from build123d import *
from build123d.topology import SkipClean

# Parameters (mm, degrees)
SKETCH3_W           = 1.5875
SKETCH3_H           = 89.802561211
BOSS_EXTRUDE2_DEPTH = 12.7
BOSS_EXTRUDE4_DEPTH = 6.35
BOSS_EXTRUDE5_DEPTH = 12.7
BOSS_EXTRUDE6_START = -6.35
BOSS_EXTRUDE6_DEPTH = 6.35
CUT_EXTRUDE1_DEPTH  = 1.5875
SKETCH5_W           = 4.7625
SKETCH5_H           = 1.5875
BOSS_EXTRUDE7_DEPTH = 70.752561211
CUT_EXTRUDE2_DEPTH  = 12.7
FILLET1_R           = 3.175
FILLET2_R           = 3.175


# Read off the part's stored shape, not the designer's step: Mirror3
with BuildPart() as part:
    # Sketch3 → Boss-Extrude2 (new body)
    with BuildSketch(Plane(origin=(0, 0, 0), x_dir=(1, 0, 0), z_dir=(0, 1, 0))):
        with Locations((0.79375, 44.901280606)):
            Rectangle(SKETCH3_W, SKETCH3_H)
    extrude(amount=BOSS_EXTRUDE2_DEPTH)

    # Sketch4 → Boss-Extrude4 (add)
    with BuildSketch(Plane(origin=(1.5875, 0, 0), x_dir=(0, 0, -1), z_dir=(1, 0, 0))):
        with BuildLine():
            ThreePointArc((0, 0), (4.490128061, 1.859871939), (6.35, 6.35))
            ThreePointArc((6.35, 6.35), (4.490128061, 10.840128061), (0, 12.7))
            Line((0, 12.7), (0, 9.525))
            ThreePointArc((0, 9.525), (2.24506403, 8.59506403), (3.175, 6.35))
            ThreePointArc((3.175, 6.35), (2.24506403, 4.10493597), (0, 3.175))
            Line((0, 3.175), (0, 0))
        make_face()
        with BuildLine():
            Line((0, 9.525), (0, 12.7))
            ThreePointArc((0, 12.7), (-6.35, 6.35), (0, 0))
            Line((0, 0), (0, 3.175))
            ThreePointArc((0, 3.175), (-3.175, 6.35), (0, 9.525))
        make_face()
        with BuildLine():
            ThreePointArc((0, 0), (4.490128061, 1.859871939), (6.35, 6.35))
            ThreePointArc((6.35, 6.35), (4.490128061, 10.840128061), (0, 12.7))
            Line((0, 12.7), (0, 9.525))
            ThreePointArc((0, 9.525), (2.24506403, 8.59506403), (3.175, 6.35))
            ThreePointArc((3.175, 6.35), (2.24506403, 4.10493597), (0, 3.175))
            Line((0, 3.175), (0, 0))
        make_face()
        with BuildLine():
            Line((0, 9.525), (0, 12.7))
            ThreePointArc((0, 12.7), (-6.35, 6.35), (0, 0))
            Line((0, 0), (0, 3.175))
            ThreePointArc((0, 3.175), (-3.175, 6.35), (0, 9.525))
        make_face()
        with BuildLine():
            Line((6.35, 0), (6.35, 6.35))
            ThreePointArc((6.35, 6.35), (4.490128061, 1.859871939), (0, 0))
            Line((0, 0), (6.35, 0))
        make_face()
        with BuildLine():
            Line((6.35, 6.35), (6.35, 12.7))
            Line((6.35, 12.7), (0, 12.7))
            ThreePointArc((0, 12.7), (4.490128061, 10.840128061), (6.35, 6.35))
        make_face()
    extrude(amount=-BOSS_EXTRUDE4_DEPTH)

    # Sketch4<6> → Boss-Extrude5 (add)
    with BuildSketch(Plane(origin=(1.5875, 0, 0), x_dir=(0, 0, -1), z_dir=(1, 0, 0))):
        Polygon((83.452561211, 12.7), (77.102561211, 12.7), (77.102561211, 0), (83.452561211, 0), (83.452561211, 6.35), align=None)
    extrude(amount=-BOSS_EXTRUDE5_DEPTH)

    # Sketch4<7> → Boss-Extrude6 (add)
    with BuildSketch(Plane(origin=(1.5875, 0, 0), x_dir=(0, 0, -1), z_dir=(1, 0, 0)).offset(BOSS_EXTRUDE6_START)):
        with BuildLine():
            ThreePointArc((89.802561211, 12.7), (85.31243315, 10.840128061), (83.452561211, 6.35))
            ThreePointArc((83.452561211, 6.35), (85.31243315, 1.859871939), (89.802561211, 0))
            Line((89.802561211, 0), (89.802561211, 3.175))
            ThreePointArc((89.802561211, 3.175), (86.627561211, 6.35), (89.802561211, 9.525))
            Line((89.802561211, 9.525), (89.802561211, 12.7))
        make_face()
        with BuildLine():
            ThreePointArc((96.152561211, 6.35), (94.292689271, 10.840128061), (89.802561211, 12.7))
            Line((89.802561211, 12.7), (89.802561211, 9.525))
            ThreePointArc((89.802561211, 9.525), (92.047625241, 8.59506403), (92.977561211, 6.35))
            ThreePointArc((92.977561211, 6.35), (92.047625241, 4.10493597), (89.802561211, 3.175))
            Line((89.802561211, 3.175), (89.802561211, 0))
            ThreePointArc((89.802561211, 0), (94.292689271, 1.859871939), (96.152561211, 6.35))
        make_face()
        with BuildLine():
            ThreePointArc((89.802561211, 12.7), (85.31243315, 10.840128061), (83.452561211, 6.35))
            ThreePointArc((83.452561211, 6.35), (85.31243315, 1.859871939), (89.802561211, 0))
            Line((89.802561211, 0), (89.802561211, 3.175))
            ThreePointArc((89.802561211, 3.175), (86.627561211, 6.35), (89.802561211, 9.525))
            Line((89.802561211, 9.525), (89.802561211, 12.7))
        make_face()
        with BuildLine():
            ThreePointArc((96.152561211, 6.35), (94.292689271, 10.840128061), (89.802561211, 12.7))
            Line((89.802561211, 12.7), (89.802561211, 9.525))
            ThreePointArc((89.802561211, 9.525), (92.047625241, 8.59506403), (92.977561211, 6.35))
            ThreePointArc((92.977561211, 6.35), (92.047625241, 4.10493597), (89.802561211, 3.175))
            Line((89.802561211, 3.175), (89.802561211, 0))
            ThreePointArc((89.802561211, 0), (94.292689271, 1.859871939), (96.152561211, 6.35))
        make_face()
        with BuildLine():
            ThreePointArc((89.802561211, 0), (85.31243315, 1.859871939), (83.452561211, 6.35))
            Line((83.452561211, 6.35), (83.452561211, 0))
            Line((83.452561211, 0), (89.802561211, 0))
        make_face()
        with BuildLine():
            Line((89.802561211, 12.7), (83.452561211, 12.7))
            Line((83.452561211, 12.7), (83.452561211, 6.35))
            ThreePointArc((83.452561211, 6.35), (85.31243315, 10.840128061), (89.802561211, 12.7))
        make_face()
    extrude(amount=-BOSS_EXTRUDE6_DEPTH)

    # Sketch4<9> → Cut-Extrude1 (cut)
    with BuildSketch(Plane(origin=(1.5875, 0, 0), x_dir=(0, 0, -1), z_dir=(1, 0, 0))):
        with BuildLine():
            ThreePointArc((89.802561211, 0), (85.31243315, 1.859871939), (83.452561211, 6.35))
            Line((83.452561211, 6.35), (83.452561211, 0))
            Line((83.452561211, 0), (89.802561211, 0))
        make_face()
        with BuildLine():
            ThreePointArc((89.802561211, 12.7), (85.31243315, 10.840128061), (83.452561211, 6.35))
            ThreePointArc((83.452561211, 6.35), (85.31243315, 1.859871939), (89.802561211, 0))
            Line((89.802561211, 0), (89.802561211, 3.175))
            ThreePointArc((89.802561211, 3.175), (86.627561211, 6.35), (89.802561211, 9.525))
            Line((89.802561211, 9.525), (89.802561211, 12.7))
        make_face()
        with BuildLine():
            ThreePointArc((96.152561211, 6.35), (94.292689271, 10.840128061), (89.802561211, 12.7))
            Line((89.802561211, 12.7), (89.802561211, 9.525))
            ThreePointArc((89.802561211, 9.525), (92.047625241, 8.59506403), (92.977561211, 6.35))
            ThreePointArc((92.977561211, 6.35), (92.047625241, 4.10493597), (89.802561211, 3.175))
            Line((89.802561211, 3.175), (89.802561211, 0))
            ThreePointArc((89.802561211, 0), (94.292689271, 1.859871939), (96.152561211, 6.35))
        make_face()
        with BuildLine():
            Line((89.802561211, 12.7), (83.452561211, 12.7))
            Line((83.452561211, 12.7), (83.452561211, 6.35))
            ThreePointArc((83.452561211, 6.35), (85.31243315, 10.840128061), (89.802561211, 12.7))
        make_face()
    extrude(amount=-CUT_EXTRUDE1_DEPTH, mode=Mode.SUBTRACT)


with BuildPart() as cut_extrude1_kept_piece:
    # of the separate pieces the step leaves, the one the design keeps (cut_extrude1_pieces_kept)
    add(part.part.solids().sort_by_distance((1.5875, 0, 0))[0])

    # Sketch5 → Boss-Extrude7 (add)
    with BuildSketch(Plane(origin=(0, 0, -6.35), x_dir=(-1, 0, 0), z_dir=(0, 0, -1))):
        with Locations((2.38125, 11.90625)):
            Rectangle(SKETCH5_W, SKETCH5_H)
        with Locations((2.38125, 0.79375)):
            Rectangle(SKETCH5_W, SKETCH5_H)
    extrude(amount=BOSS_EXTRUDE7_DEPTH)

    # Sketch4<10> → Cut-Extrude2 (cut)
    with SkipClean():  # the faces are left unmerged after this step: merging them gives an invalid solid
        with BuildSketch(Plane(origin=(1.5875, 0, 0), x_dir=(0, 0, -1), z_dir=(1, 0, 0))):
            with BuildLine():
                ThreePointArc((3.175, 6.35), (2.24506403, 8.59506403), (0, 9.525))
                Line((0, 9.525), (0, 3.175))
                ThreePointArc((0, 3.175), (2.24506403, 4.10493597), (3.175, 6.35))
            make_face()
            with BuildLine():
                Line((0, 3.175), (0, 9.525))
                ThreePointArc((0, 9.525), (-3.175, 6.35), (0, 3.175))
            make_face()
        extrude(amount=-CUT_EXTRUDE2_DEPTH, mode=Mode.SUBTRACT)

    # Fillet1
    fillet1_edges = [cut_extrude1_kept_piece.edges().sort_by_distance(p)[0] for p in [
        (0, 6.35, -77.102561211),
    ]]
    fillet(fillet1_edges, radius=FILLET1_R)

    # Fillet2
    fillet2_edges = [cut_extrude1_kept_piece.edges().sort_by_distance(p)[0] for p in [
        (0, 6.35, -6.35),
    ]]
    fillet(fillet2_edges, radius=FILLET2_R)

    # Mirror3: Cut-Extrude1 kept piece across plane


with BuildPart() as cut_extrude1_kept_piece_1:
    with SkipClean():  # the faces are left unmerged after this step: merging them gives an invalid solid
        add(cut_extrude1_kept_piece.part)
        add(cut_extrude1_kept_piece.part.mirror(Plane(origin=(1.5875, 0, 0), x_dir=(0, 0, 1), z_dir=(1, 0, 0))))


solid = cut_extrude1_kept_piece_1.part
CAD build for the part. Positions are in the model's coordinates, mm. A direction names the side the tool comes from. Round coordinates to 2 decimals unless told otherwise and drop trailing zeros. Loops run counter-clockwise (first coordinate to the right, second up) from the corner with the lowest first, then second, coordinate; pieces in that order, holes last.
(1) Cut at B-B (z = -69). Give the cut face in (x, y) (1 decimal).
(2) Cut at A-A (x = 10.5). Give the cut face in (y, z) (3 decimals), plus the area to 3 significant figures.
(3) Cut at C-C (y = 8). State how many separate pieces and enclosed holes the cut face has, plus the area to 3 significant figures.
(4) Wall check: line 1 along Y through (x, z) = (5.75, 0) (3 decimals); line 2 along Y through (x, z) = (-4.5, -39.5); line 3 along Z through (x, y) = (5.5, 5.5). Give the ranges that are in metal, low to high.
(5) Which spindle directions (+Z, -Z, +X, -X, +Y, -Y) get a long thin tool onto all of the face, cutting with end or side? Do faces 1 (the flat face through (7.938, 4, -87)), 2 (the flat face through (6, 1.588, -41)), 3 (the flat face through (-4.762, 1, -32)), 4 (the flat face through (-2, 11.112, -41)). Say none if no direction does.
(6) Two-plate mould, pull along Y, no slides. Class faces 5 (the flat face through (7.938, 1, -32)), 6 (the cylindrical face through (4.08, 6.283, -7.305)), 7 (the flat face through (1, 12.7, -44)): +Y half, -Y half, draft (parallel to the pull), parting line (faces both ways), or undercut.
(7) Drop flat-ended pins along their axis: pin 1 (2.5 mm diameter, centred on x = -7.5, y = 6.5, fed in from +Z); pin 2 (2 mm diameter, centred on x = -3, y = 9, fed in from +Z); pin 3 (5 mm diameter, centred on x = -2.5, z = -40, fed in from -Y); pin 4 (1.9 mm diameter, centred on x = 6, y = 4.5, fed in from -Z). Give the stop position or say it passes through.
Findings below:
1. outline: (-4.8, 0) - (7.9, 0) - (7.9, 1.6) - (3.2, 1.6) - (3.2, 11.1) - (7.9, 11.1) - (7.9, 12.7) - (-4.8, 12.7) - (-4.8, 11.1) - (0, 11.1) - (0, 1.6) - (-4.8, 1.6) - close
2. outline: (0, -89.803) arc R6.35 ccw to (12.7, -89.803) - (12.7, -77.103) - (0, -77.103) - close; hole circle Ø6.35 at (6.35, -89.803)
2. area: 193 mm2
3. separate pieces: 4
3. enclosed holes: 0
3. area: 574 mm2
4. line 1: y = 0 to 3.175, 9.525 to 12.7
4. line 2: y = 0 to 1.59, 11.11 to 12.7
4. line 3: z = -83.45 to -76.99, -6.47 to -3.06, 3.06 to 6.29
5. face 1: -Z, +Y, -Y
5. face 2: +X
5. face 3: +Z, -X, +Y, -Y
5. face 4: -X
6. face 5: draft
6. face 6: undercut
6. face 7: +Y half
7. pin 1: stops at z = -77.1
7. pin 2: stops at z = 6.13
7. pin 3: stops at y = 0
7. pin 4: stops at z = -83.45
